Geometry check sheet. Reference: drawing and pictorial views, mm from the part's lowest x, y, z. A direction names the side the tool comes from. Coordinates: 2 decimals unless noted, no trailing zeros. Order: outer loops, then holes, each group sorted by start corner. A loop starts at its lowest first (then second) coordinate and runs counter-clockwise, first axis right, second up. Notation, with made-up numbers: (88.5, 80) -> (141.5, 80) arc R10 cw to (141.5, 98) -> close; hole circle Ø7 at (-10.5, 39.25). An arc over 180 degrees is marked (long way). Use CSV: the item, a comma, the result in double quotes. Start each with the question number.
1) Scan lines: line 1 along X through (y, z) = (60, 4); line 2 along X through (y, z) = (60, 12.5). Record each from-to range of solid material in increasing order.
2) Sectioned sample at B-B on y = 20. Record the boundary of the cut face in (x, z), then the cut area to 3 significant figures.
3) Tool access check on the marked faces 1 and 2. Record the directions out of +Z, -Z, +X, -X, +Y, -Y that give a thin tool (end or side, any length) a straight path to the whole face; none if there is none.
4) Sectioned sample at D-D on z = 1.75. Record the boundary of the cut face in (x, y).
5) Go/stop test with flat-tipped pins: pin 1 (7.5 mm diameter, centred on x = 20, y = 60, fed in from +Z); pin 2 (12 mm diameter, centred on x = 20, y = 20, fed in from +Z). Record where each tip stops, or that it passes through.
6) Sectioned sample at A-A on z = 9.75. Record the boundary of the cut face in (x, y), then the cut area to 3 significant figures.
7) Release check for a two-part mould opening along Y. For the marked faces 3, 4, 5 and 6 record: released by +Y, released by -Y, zero draft, split by the parting line, or undercut.
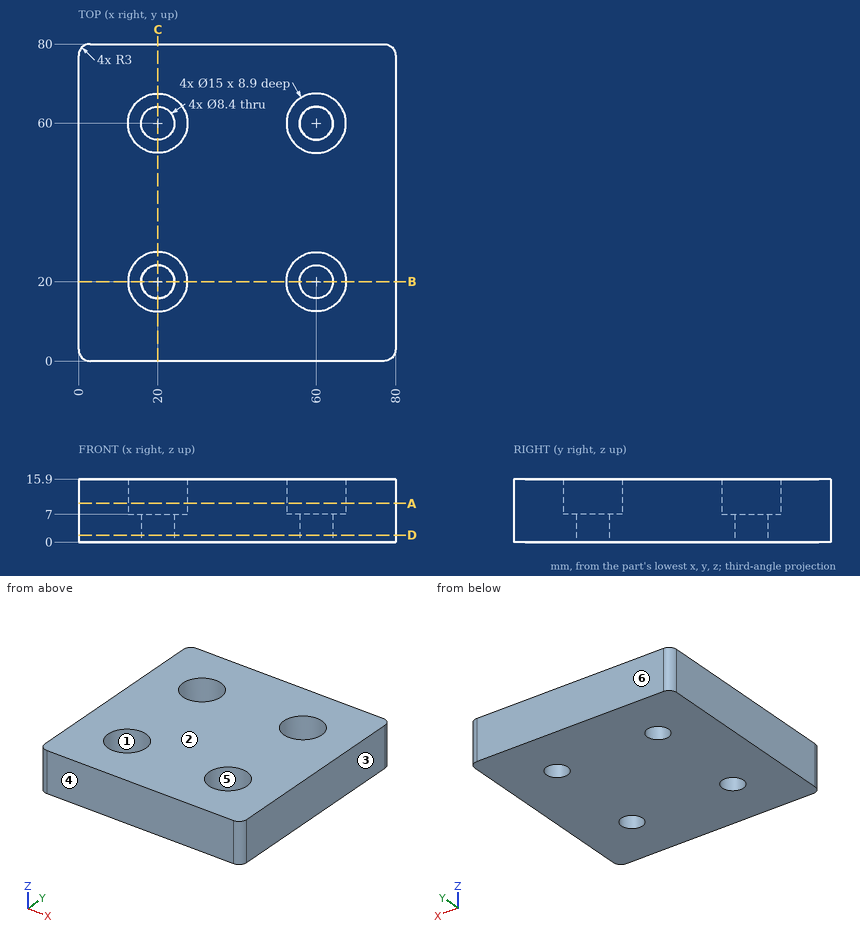
Answers follow:
1,line 1,"x = 0 to 15.8, 24.2 to 55.8, 64.2 to 80"
1,line 2,"x = 0 to 12.5, 27.5 to 52.5, 67.5 to 80"
2,outline,"(0, 0) -> (15.8, 0) -> (15.8, 7) -> (12.5, 7) -> (12.5, 15.9) -> (0, 15.9) -> close; (24.2, 0) -> (55.8, 0) -> (55.8, 7) -> (52.5, 7) -> (52.5, 15.9) -> (27.5, 15.9) -> (27.5, 7) -> (24.2, 7) -> close; (64.2, 0) -> (80, 0) -> (80, 15.9) -> (67.5, 15.9) -> (67.5, 7) -> (64.2, 7) -> close"
2,area,"887 mm²"
3,face 1,"+Z"
3,face 2,"+Z, +X, -X, +Y, -Y"
4,outline,"(0, 3) arc R3 ccw to (3, 0) -> (77, 0) arc R3 ccw to (80, 3) -> (80, 77) arc R3 ccw to (77, 80) -> (3, 80) arc R3 ccw to (0, 77) -> close; hole circle Ø8.4 at (20, 20); hole circle Ø8.4 at (20, 60); hole circle Ø8.4 at (60, 20); hole circle Ø8.4 at (60, 60)"
5,pin 1,"passes through"
5,pin 2,"stops at z = 7"
6,outline,"(0, 3) arc R3 ccw to (3, 0) -> (77, 0) arc R3 ccw to (80, 3) -> (80, 77) arc R3 ccw to (77, 80) -> (3, 80) arc R3 ccw to (0, 77) -> close; hole circle Ø15 at (20, 20); hole circle Ø15 at (20, 60); hole circle Ø15 at (60, 20); hole circle Ø15 at (60, 60)"
6,area,"5,690 mm²"
7,face 3,"zero draft"
7,face 4,"released by -Y"
7,face 5,"undercut"
7,face 6,"released by +Y"
